from build123d import *

# Parameters (mm, degrees)
SKETCH1_W           = 39.25
SKETCH1_H           = 24.25
BOSS_EXTRUDE1_DEPTH = 1.5
SKETCH2_W           = 42.75
SKETCH2_H           = 30.25
SKETCH2_W_2         = 39.25
SKETCH2_H_2         = 24.25
BOSS_EXTRUDE2_DEPTH = 18.5
SKETCH3_W           = 2
SKETCH3_H           = 8
CUT_EXTRUDE1_DEPTH  = 10.8
CUT_EXTRUDE2_REACH  = 44.75
CUT_EXTRUDE3_DEPTH  = 14
SKETCH7_R           = 1
CUT_EXTRUDE4_DEPTH  = 2.5


with BuildPart() as part:
    # Sketch1 → Boss-Extrude1 (new body)
    with BuildSketch(Plane(origin=(0, 0, 0), x_dir=(1, 0, 0), z_dir=(0, 1, 0))):
        Rectangle(SKETCH1_W, SKETCH1_H)
    extrude(amount=BOSS_EXTRUDE1_DEPTH)

    # Sketch2 → Boss-Extrude2 (add)
    with BuildSketch(Plane(origin=(0, 0, 0), x_dir=(1, 0, 0), z_dir=(0, 1, 0))):
        with Locations((-0.25, 0)):
            Rectangle(SKETCH2_W, SKETCH2_H)
        Rectangle(SKETCH2_W_2, SKETCH2_H_2, mode=Mode.SUBTRACT)
    extrude(amount=BOSS_EXTRUDE2_DEPTH)

    # Sketch3 → Cut-Extrude1 (cut)
    with BuildSketch(Plane(origin=(0, 18.5, 0), x_dir=(1, 0, 0), z_dir=(0, 1, 0))):
        with Locations((-20.625, -3.125)):
            Rectangle(SKETCH3_W, SKETCH3_H)
    extrude(amount=-CUT_EXTRUDE1_DEPTH, mode=Mode.SUBTRACT)

    # Sketch4 → Cut-Extrude2 (cut, up to next)
    with BuildSketch(Plane(origin=(21.125, 0, 0), x_dir=(0, 0, -1), z_dir=(1, 0, 0)), mode=Mode.PRIVATE) as cut_extrude2_sk1:
        with BuildLine():
            Line((-3.625, 14.5), (3.625, 14.5))
            ThreePointArc((3.625, 14.5), (4.332106781, 14.792893219), (4.625, 15.5))
            Line((4.625, 15.5), (4.625, 16.75))
            ThreePointArc((4.625, 16.75), (4.332106781, 17.457106781), (3.625, 17.75))
            Line((3.625, 17.75), (-3.625, 17.75))
            ThreePointArc((-3.625, 17.75), (-4.332106781, 17.457106781), (-4.625, 16.75))
            Line((-4.625, 16.75), (-4.625, 15.5))
            ThreePointArc((-4.625, 15.5), (-4.332106781, 14.792893219), (-3.625, 14.5))
        make_face()
    cut_extrude2_tool1 = extrude(cut_extrude2_sk1.sketch, amount=-CUT_EXTRUDE2_REACH, mode=Mode.PRIVATE) & part.part
    add(cut_extrude2_tool1.solids().sort_by_distance((21.125, 16.125, 0))[0], mode=Mode.SUBTRACT)

    # Sketch6 → Cut-Extrude3 (cut)
    with BuildSketch(Plane(origin=(0, 18.5, 0), x_dir=(1, 0, 0), z_dir=(0, 1, 0))):
        Polygon((-5, 15.125), (-7.598076211, 13.625), (-5, 12.125), (5, 12.125), (7.598076211, 13.625), (5, 15.125), align=None)
        Polygon((-7.598076211, -13.625), (-5, -12.125), (5, -12.125), (7.598076211, -13.625), (5, -15.125), (-5, -15.125), align=None)
    extrude(amount=-CUT_EXTRUDE3_DEPTH, mode=Mode.SUBTRACT)

    # Sketch7 → Cut-Extrude4 (cut, through all)
    with BuildSketch(Plane(origin=(0, 1.5, 0), x_dir=(1, 0, 0), z_dir=(0, 1, 0))):
        with Locations((-16.025, -6.875)):
            Circle(SKETCH7_R)
        with Locations((-16.025, -4.335)):
            Circle(SKETCH7_R)
        with Locations((-16.025, -1.795)):
            Circle(SKETCH7_R)
        with Locations((-16.025, 0.745)):
            Circle(SKETCH7_R)
        with Locations((-16.025, 3.285)):
            Circle(SKETCH7_R)
        with Locations((-16.025, 5.825)):
            Circle(SKETCH7_R)
    extrude(amount=-CUT_EXTRUDE4_DEPTH, mode=Mode.SUBTRACT)


solid = part.part
Read the model definition and answer for the solid it produces. Units are mm, in the model's axes. A direction names the side the tool comes from. Give positions to 0.01 mm unless a question says otherwise; leave off trailing zeros. Write each loop counter-clockwise with the first axis right and the second up, starting at its lowest first coordinate (ties: lowest second). Pieces come first, ordered by that corner, then holes. Notation, with made-up numbers: (69.25, 19) - (93.25, 19) arc R6 cw to (93.25, 30) - close; hole circle Ø10 at (29, 51). An arc over 180 degrees is marked (long way). Return JSON: item names as keys, results as strings.
Q1. A cutting plane is placed at D-D, the plane z = -10. Determine the outline of the cut face in (x, y) (3 decimals).
Reply:
{"outline": "(-21.625, 0) - (21.125, 0) - (21.125, 18.5) - (19.625, 18.5) - (19.625, 1.5) - (-19.625, 1.5) - (-19.625, 18.5) - (-21.625, 18.5) - close"}
Q2. A cutting plane is placed at A-A, the plane y = 4. Determine the outline of the cut face in (x, z) (3 decimals).
Reply:
{"outline": "(-21.625, -15.125) - (21.125, -15.125) - (21.125, 15.125) - (-21.625, 15.125) - close; hole (-19.625, -12.125) - (19.625, -12.125) - (19.625, 12.125) - (-19.625, 12.125) - close"}
Q3. Consider line 1 along X through (y, z) = (1.75, -11) (3 decimals); line 2 along Z through (x, y) = (-7.5, 2.25) (3 decimals); line 3 along Y through (x, z) = (4, -2). Determine where each line is inside the solid, lowest interval first. Write a range as [from, to].
Reply:
{"line 1": "[-21.625, -19.625], [19.625, 21.125]", "line 2": "[-15.125, -12.125], [12.125, 15.125]", "line 3": "[0, 1.5]"}
Q4. A cutting plane is placed at C-C, the plane y = 12.75. Determine the outline of the cut face in (x, z) (3 decimals), and give its area (3 significant figures).
Reply:
{"outline": "(-21.625, -15.125) - (-5, -15.125) - (-7.598, -13.625) - (-5, -12.125) - (-19.625, -12.125) - (-19.625, -0.875) - (-21.625, -0.875) - close; (-21.625, 7.125) - (-19.625, 7.125) - (-19.625, 12.125) - (-5, 12.125) - (-7.598, 13.625) - (-5, 15.125) - (-21.625, 15.125) - close; (5, -15.125) - (21.125, -15.125) - (21.125, 15.125) - (5, 15.125) - (7.598, 13.625) - (5, 12.125) - (19.625, 12.125) - (19.625, -12.125) - (5, -12.125) - (7.598, -13.625) - close", "area": "250 mm²"}
Q5. For faces 4 (the face through (20.39, 14.8, 4.34)), 5 (the face through (20.39, 17.45, -4.34)), 6 (the face through (-21, 13, 7.125)), 7 (the face through (-6.317, 11.598, 12.886)), determine the directions among +Z, -Z, +X, -X, +Y, -Y from which every point of the face is accessible in a straight line to the end or side of a thin tool.
Reply:
{"face 4": "+X, -X", "face 5": "+X", "face 6": "-X, +Y", "face 7": "+Y"}
Q6. Given P1, Ø6, axis at x = 13.5, z = 3.5, coming from the +Y side; P2, Ø1.8, axis at x = -16.025, z = -3.285, coming from the +Y side; P3, Ø3.5, axis at x = -0.5, z = -14.5, coming from the +Y side, each flat-ended and moving along its own axis, determine where each tip first touches the part or whether it passes through.
Reply:
{"P1": "y = 1.5", "P2": "through", "P3": "y = 4.5"}
Q7. A cutting plane is placed at B-B, the plane x = -14.5. Determine the outline of the cut face in (y, z) (3 decimals), and give its area (3 significant figures).
Reply:
{"outline": "(0, -15.125) - (18.5, -15.125) - (18.5, -12.125) - (1.5, -12.125) - (1.5, 12.125) - (18.5, 12.125) - (18.5, 15.125) - (0, 15.125) - close", "area": "147 mm²"}
Q8. For a pull along Y with two mould halves and no side action, classify faces 1 (the face through (-15.071, 0.76, -1.045)), 2 (the face through (20.386, 14.785, -4.324)), 3 (the face through (-16.4, 18.5, -12.3)) as released by +Y, released by -Y, zero draft, split by the parting line, or undercut.
Reply:
{"face 1": "zero draft", "face 2": "undercut", "face 3": "released by +Y"}
